Input: part model. Units: mm. Frame: model coordinates. Give positions to 0.01 mm unless a question says otherwise; leave off trailing zeros. Order: outer loops, then holes, each group sorted by start corner. A loop starts at its lowest first (then second) coordinate and runs counter-clockwise, first axis right, second up. Notation, with made-up numbers: M 79,-37.75 L 90,-37.75 A27 ccw 90,-8.75 Z; hole C 85,31 d10. An arc over 180 degrees is marked long. Use a Markdown table: item, result.
from build123d import *

# Parameters (mm, degrees)
SKETCH1_R                      = 152.4
BOSS_EXTRUDE1_DEPTH            = 6.35
M5X0_8_SET_SCREWS_D            = 4.2
SKETCH5_R                      = 3.175
CUT_EXTRUDE1_DEPTH             = 7.35
CIRPATTERN1_COUNT              = 6
SKETCH6_R                      = 12.7
CUT_EXTRUDE2_DEPTH             = 7.35
CBORE_FOR_M4_SHCS1_D           = 4.5
CBORE_FOR_M4_SHCS1_CBORE_D     = 8
CBORE_FOR_M4_SHCS1_CBORE_DEPTH = 6


with BuildPart() as part:
    # Sketch1 → Boss-Extrude1 (new body)
    with BuildSketch(Plane(origin=(0, 0, 0), x_dir=(1, 0, 0), z_dir=(0, 1, 0))):
        Circle(SKETCH1_R)
    extrude(amount=BOSS_EXTRUDE1_DEPTH)

    # M5x0.8 Set Screws (through all)
    with Locations(Plane(origin=(0, 6.35, 0), x_dir=(1, 0, 0), z_dir=(0, 1, 0))):
        with Locations((-38.494829198, 127.225), (38.494829198, 127.225), (0, 60.55)):
            m5x0_8_set_screws = Hole(M5X0_8_SET_SCREWS_D / 2)

    # Sketch5 → Cut-Extrude1 (cut, through all)
    with BuildSketch(Plane(origin=(0, 6.35, 0), x_dir=(1, 0, 0), z_dir=(0, 1, 0))):
        with Locations((0, 105)):
            Circle(SKETCH5_R)
    cut_extrude1 = extrude(amount=-CUT_EXTRUDE1_DEPTH, mode=Mode.SUBTRACT)

    # CirPattern1: M5x0.8 Set Screws, Cut-Extrude1 ×6 about axis
    cirpattern1_axis = Axis((0, 0, 0), (0, 1, 0))
    for i in range(1, CIRPATTERN1_COUNT):
        add(m5x0_8_set_screws.rotate(cirpattern1_axis, i * 360 / CIRPATTERN1_COUNT), mode=Mode.SUBTRACT)
        add(cut_extrude1.rotate(cirpattern1_axis, i * 360 / CIRPATTERN1_COUNT), mode=Mode.SUBTRACT)

    # Sketch6 → Cut-Extrude2 (cut, through all)
    with BuildSketch(Plane(origin=(0, 6.35, 0), x_dir=(1, 0, 0), z_dir=(0, 1, 0))):
        Circle(SKETCH6_R)
    extrude(amount=-CUT_EXTRUDE2_DEPTH, mode=Mode.SUBTRACT)

    # CBORE for M4 SHCS1 (through all)
    with Locations(Plane(origin=(0, 6.35, 0), x_dir=(1, 0, 0), z_dir=(0, 1, 0))):
        with Locations((-15.0260191, 15.0260191), (15.0260191, 15.0260191), (15.0260191, -15.0260191), (-15.0260191, -15.0260191)):
            CounterBoreHole(CBORE_FOR_M4_SHCS1_D / 2, CBORE_FOR_M4_SHCS1_CBORE_D / 2, CBORE_FOR_M4_SHCS1_CBORE_DEPTH)


solid = part.part
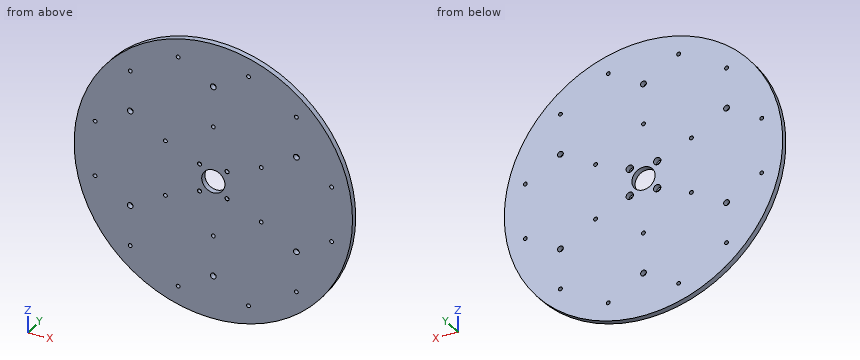
1) Material intervals for line 1 (Z direction, x = -130, y = 2.5); line 2 (X direction, y = 3, z = 0); line 3 (Z direction, x = 11.5, y = 4), sorted ascending. Write a range as from..to.
Response values:
| item | result |
|---|---|
| line 1 | z = -79.53..-32.3, -28.25..28.25, 32.3..79.53 |
| line 2 | x = -152.4..-12.7, 12.7..152.4 |
| line 3 | z = -151.97..-16.91, -13.14..-5.39, 5.39..13.14, 16.91..151.97 |
2) Cut plane C-C on x = 108. Return loops of the section in (y, z).
Response values:
| item | result |
|---|---|
| outline | M 0,-107.53 L 6.35,-107.53 L 6.35,107.53 L 0,107.53 Z |
3) First-contact query: pin 1 Ø4 at (x, z) = (16, -15.5) entering from +Y; pin 2 Ø3 at (y, z) = (1.5, 43.5) entering from -X; pin 3 Ø2 at (y, z) = (5.5, -104) entering from +X. Flat tips, straight axial feed; report the tip coordinate or a pass-through.
Response values:
| item | result |
|---|---|
| pin 1 | stops at y = 0.35 |
| pin 2 | stops at x = -146.5 |
| pin 3 | stops at x = 112.32 |
4) Cut plane A-A on z = 0. Return loops of the section in (x, y), and give its area (3 significant figures).
Response values:
| item | result |
|---|---|
| outline | M -152.4,0 L -12.7,0 L -12.7,6.35 L -152.4,6.35 Z; M 12.7,0 L 152.4,0 L 152.4,6.35 L 12.7,6.35 Z |
| area | 1,770 mm² |
5) Cut plane B-B on y = 3.5. State how many separate pieces and enclosed holes the cut face has, and give its area (3 significant figures).
Response values:
| item | result |
|---|---|
| separate pieces | 1 |
| enclosed holes | 29 |
| area | 71,800 mm² |
